Source: CAD feature listing. Evaluate the final solid. Frame: model axes, mm. A direction names the side the tool comes from. Coordinates: 2 decimals unless noted, no trailing zeros. Order: outer loops, then holes, each group sorted by start corner. A loop starts at its lowest first (then second) coordinate and runs counter-clockwise, first axis right, second up.
```python
from build123d import *

# Parameters (mm, degrees)
CHAMFER_1_SIZE                 = 0.5
CHAMFER_2_SIZE                 = 0.2
HOLE_WIZARD_6_0_6_1_AT_2_COUNT = 2
HOLE_WIZARD_6_0_6_1_AT_2_PITCH = 48
HOLE_WIZARD_6_0_6_1_AT_3_COUNT = 2
HOLE_WIZARD_6_0_6_1_AT_3_PITCH = 113
HOLE_WIZARD_6_0_6_1_AT_4_COUNT = 2
HOLE_WIZARD_6_0_6_1_AT_4_PITCH = 161
PATTERN_CIRCULAR_1_COUNT       = 2
PATTERN_CIRCULAR_1_ANGLE       = 90
CUT_EXTRUDE_3_DEPTH            = 10
HOLE_WIZARD_M4_1_D             = 3.3
HOLE_WIZARD_M4_1_DEPTH         = 11.5
HOLE_WIZARD_M4_1_TIP           = 0.991420021


with BuildPart() as part:
    # 草图1 → 旋转1 (revolve)
    with BuildSketch(Plane.XY):
        Polygon((0, 0), (0, -239.5), (-7.5, -239.5), (-7.5, -233.5), (-9, -233.5), (-9, -33.5), (-7.5, -33.5), (-7.5, -28.5), (-5, -28.5), (-5, 0), align=None)
    revolve(axis=Axis((0, 0, 0), (0, -1, 0)))

    # 倒角1
    chamfer_1_edges = [part.edges().sort_by_distance(p)[0] for p in [
        (7.5, -239.5, 0),
        (5, 0, 0),
        (7.5, -28.5, 0),
    ]]
    chamfer(chamfer_1_edges, length=CHAMFER_1_SIZE)

    # 倒角2
    chamfer_2_edges = [part.edges().sort_by_distance(p)[0] for p in [
        (9, -33.5, 0),
        (9, -233.5, 0),
    ]]
    chamfer(chamfer_2_edges, length=CHAMFER_2_SIZE)

    # 草图5 → Ø6.0 (6) 直径孔1 (revolve, cut)
    with BuildSketch(Plane(origin=(0, -214, -9), x_dir=(0, 1, 0), z_dir=(1, 0, 0))):
        Polygon((0, 0), (0, 3.802581857), (3, 2), (3, 0), align=None)
    hole_wizard_6_0_6_1 = revolve(axis=Axis((0, -214, -15.35), (0, 0, 1)), mode=Mode.SUBTRACT)

    # Ø6.0 (6) 直径孔1 at 2: Ø6.0 (6) 直径孔1 ×2
    with Locations(*[(0, i * HOLE_WIZARD_6_0_6_1_AT_2_PITCH, 0) for i in range(1, HOLE_WIZARD_6_0_6_1_AT_2_COUNT)]):
        add(hole_wizard_6_0_6_1, mode=Mode.SUBTRACT)

    # Ø6.0 (6) 直径孔1 at 3: Ø6.0 (6) 直径孔1 ×2
    with Locations(*[(0, i * HOLE_WIZARD_6_0_6_1_AT_3_PITCH, 0) for i in range(1, HOLE_WIZARD_6_0_6_1_AT_3_COUNT)]):
        add(hole_wizard_6_0_6_1, mode=Mode.SUBTRACT)

    # Ø6.0 (6) 直径孔1 at 4: Ø6.0 (6) 直径孔1 ×2
    with Locations(*[(0, i * HOLE_WIZARD_6_0_6_1_AT_4_PITCH, 0) for i in range(1, HOLE_WIZARD_6_0_6_1_AT_4_COUNT)]):
        add(hole_wizard_6_0_6_1, mode=Mode.SUBTRACT)

    # 阵列(圆周)1: Ø6.0 (6) 直径孔1 ×2 about axis
    pattern_circular_1_axis = Axis((0, 0, 0), (0, 1, 0))
    for i in range(1, PATTERN_CIRCULAR_1_COUNT):
        add(hole_wizard_6_0_6_1.rotate(pattern_circular_1_axis, i * PATTERN_CIRCULAR_1_ANGLE / (PATTERN_CIRCULAR_1_COUNT - 1)), mode=Mode.SUBTRACT)

    # 阵列(圆周)1 copy 1 sketch → 阵列(圆周)1 copy 1 (revolve, cut)
    with BuildSketch(Plane(origin=(-9, -166, 0), x_dir=(0, 1, 0), z_dir=(0, 0, -1))):
        Polygon((0, 0), (0, 3.802581857), (3, 2), (3, 0), align=None)
    revolve(axis=Axis((-15.35, -166, 0), (1, 0, 0)), mode=Mode.SUBTRACT)

    # 阵列(圆周)1 copy 2 sketch → 阵列(圆周)1 copy 2 (revolve, cut)
    with BuildSketch(Plane(origin=(-9, -101, 0), x_dir=(0, 1, 0), z_dir=(0, 0, -1))):
        Polygon((0, 0), (0, 3.802581857), (3, 2), (3, 0), align=None)
    revolve(axis=Axis((-15.35, -101, 0), (1, 0, 0)), mode=Mode.SUBTRACT)

    # 阵列(圆周)1 copy 3 sketch → 阵列(圆周)1 copy 3 (revolve, cut)
    with BuildSketch(Plane(origin=(-9, -53, 0), x_dir=(0, 1, 0), z_dir=(0, 0, -1))):
        Polygon((0, 0), (0, 3.802581857), (3, 2), (3, 0), align=None)
    revolve(axis=Axis((-15.35, -53, 0), (1, 0, 0)), mode=Mode.SUBTRACT)

    # 草图7 → 切除-拉伸3 (cut)
    with BuildSketch(Plane.XY.offset(2.5)):
        with BuildLine():
            Line((2, -5), (2, -15))
            ThreePointArc((2, -15), (0, -17), (-2, -15))
            Line((-2, -15), (-2, -5))
            ThreePointArc((-2, -5), (0, -3), (2, -5))
        make_face()
    extrude(amount=CUT_EXTRUDE_3_DEPTH, mode=Mode.SUBTRACT)

    # M4 螺纹孔1
    with Locations(Plane(origin=(0, 0, 0), x_dir=(1, 0, 0), z_dir=(0, 1, 0))):
        with Locations((0, 0)):
            Hole(HOLE_WIZARD_M4_1_D / 2, depth=HOLE_WIZARD_M4_1_DEPTH)
            with Locations((0, 0, -(HOLE_WIZARD_M4_1_DEPTH + HOLE_WIZARD_M4_1_TIP / 2))):  # 118° drill point
                Cone(0, HOLE_WIZARD_M4_1_D / 2, HOLE_WIZARD_M4_1_TIP, mode=Mode.SUBTRACT)


solid = part.part
```
1. Pin query (flat end, axial travel): P1, Ø4, axis at y = -68, z = -4, coming from the +X side; P2, Ø5.5, axis at y = -53, z = 0, coming from the -X side; P3, Ø4, axis at x = 2.5, z = -6.5, coming from the +Y side. Return the tip coordinate at first contact, or that it passes through.
Findings:
P1: stops at x = 8.77
P2: stops at x = -6.85
P3: stops at y = -0.46
2. Draft query along Z for faces 5 (the face through (-5.5, -214.5, 0)), 6 (the face through (0, -214.5, -5.5)), 7 (the face through (0, -10, 2.5)), 8 (the face through (-3, -14, -4)). Return one class per face: released by +Z, released by -Z, zero draft, split by the parting line, or undercut.
Findings:
face 5: undercut
face 6: released by -Z
face 7: released by +Z
face 8: split by the parting line
3. Access query for faces 1 (the face through (7.493, -236.212, -0.33)), 2 (the face through (1.15, -98.23, -7.79)), 3 (the face through (-7.79, -211.14, 0.9)), 4 (the face through (7.493, -31.218, -0.33)). Directions: +Z, -Z, +X, -X, +Y, -Y. A direction counts if a zero-diameter tool reaches every point of the face in a straight line with its end or side. Return the directions, or none.
Findings:
face 1: -Y
face 2: -Z
face 3: -X
face 4: +Y
4. Section query A-A on y = -46. Return loops of the section in (x, z).
Findings:
outline: circle Ø18 at (0, 0)
5. Ray query, line 1 (Y direction, x = 0, z = -7.85); line 2 (Z direction, x = 0, y = -2.5); line 3 (Z direction, x = 4, y = -26). Return the intervals inside material, ascending.
Findings:
line 1: y = -233.5 to -217, -211 to -169, -163 to -104, -98 to -56, -50 to -33.5
line 2: z = -5 to -1.65, 1.65 to 5
line 3: z = -3 to 3
